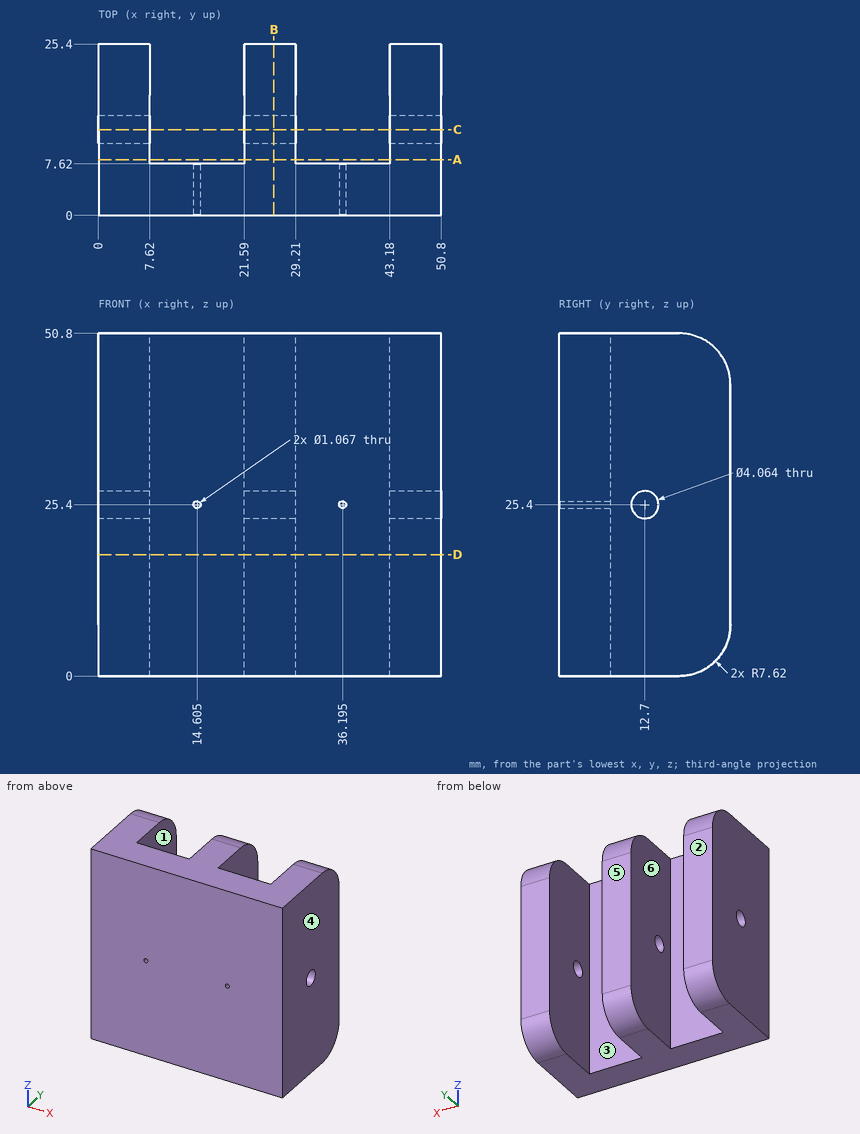
Can you work these out from the drawing? Everything is in mm from the part's minimum corner. A direction names the side the tool comes from. Round coordinates to 2 decimals unless told otherwise and drop trailing zeros. Write each loop counter-clockwise with the first axis right and the second up, starting at its lowest first coordinate (ties: lowest second). Pieces come first, ordered by that corner, then holes. Notation, with made-up numbers: (-1.75, 73.25) - (50.25, 73.25) arc R16 ccw to (50.25, 88.25) - close; hole circle Ø9 at (-29, 78). An arc over 180 degrees is marked (long way). Use a Markdown table: item, result.
Q1. I want a section at B-B (x = 26). List the corners of the cut face in (y, z) for me.
Output values:
| item | result |
|---|---|
| outline | (0, 0) - (17.78, 0) arc R7.62 ccw to (25.4, 7.62) - (25.4, 43.18) arc R7.62 ccw to (17.78, 50.8) - (0, 50.8) - close; hole circle Ø4.06 at (12.7, 25.4) |
Q2. I want a section at C-C (y = 12.7). List the corners of the cut face in (x, z) for me, plus the area to 3 significant figures.
Output values:
| item | result |
|---|---|
| outline | (0, 0) - (7.62, 0) - (7.62, 23.37) - (0, 23.37) - close; (0, 27.43) - (7.62, 27.43) - (7.62, 50.8) - (0, 50.8) - close; (21.59, 0) - (29.21, 0) - (29.21, 23.37) - (21.59, 23.37) - close; (21.59, 27.43) - (29.21, 27.43) - (29.21, 50.8) - (21.59, 50.8) - close; (43.18, 0) - (50.8, 0) - (50.8, 23.37) - (43.18, 23.37) - close; (43.18, 27.43) - (50.8, 27.43) - (50.8, 50.8) - (43.18, 50.8) - close |
| area | 1,070 mm2 |
Q3. I want a section at D-D (z = 18). List the corners of the cut face in (x, y) for me.
Output values:
| item | result |
|---|---|
| outline | (0, 0) - (50.8, 0) - (50.8, 25.4) - (43.18, 25.4) - (43.18, 7.62) - (29.21, 7.62) - (29.21, 25.4) - (21.59, 25.4) - (21.59, 7.62) - (7.62, 7.62) - (7.62, 25.4) - (0, 25.4) - close |
Q4. For the marked faces 1 and 2, which set-ups out of +Z, -Z, +X, -X, +Y, -Y let a thin tool reach every point of the face, with its end or its side?
Output values:
| item | result |
|---|---|
| face 1 | +Z, -Z, +Y |
| face 2 | +Z, -Z, +X, -X, +Y |
Q5. I want a section at A-A (y = 8.25). List the corners of the cut face in (x, z) for me.
Output values:
| item | result |
|---|---|
| outline | (0, 0) - (7.62, 0) - (7.62, 50.8) - (0, 50.8) - close; (21.59, 0) - (29.21, 0) - (29.21, 50.8) - (21.59, 50.8) - close; (43.18, 0) - (50.8, 0) - (50.8, 50.8) - (43.18, 50.8) - close |
Q6. Please list where these lines run through material, in increasing order: L1, parallel to X at y = 10.25, z = 36; L2, parallel to Z at x = 47.5, y = 12.7; L3, parallel to Y at x = 32, z = 32.
Output values:
| item | result |
|---|---|
| L1 | 0 to 7.62, 21.59 to 29.21, 43.18 to 50.8 |
| L2 | 0 to 23.37, 27.43 to 50.8 |
| L3 | 0 to 7.62 |
Q7. For pin 1 (4 mm diameter, centred on x = 34.5, z = 13.5, fed in from +Y); pin 2 (0.6 mm diameter, centred on x = 36.195, z = 25.4, fed in from -Y), each with a flat end and sliding along its axis, tell me the tip position at first contact or that it passes through.
Output values:
| item | result |
|---|---|
| pin 1 | y = 7.62 |
| pin 2 | through |
Q8. Thinking about a two-plate mould opening in X: for the marked faces 3, 4, 5 and 6, which applies, released by +X, released by -X, zero draft, split by the parting line, or undercut?
Output values:
| item | result |
|---|---|
| face 3 | undercut |
| face 4 | released by +X |
| face 5 | zero draft |
| face 6 | undercut |
